from build123d import *

# Parameters (mm, degrees)
CUT_EXTRUDE1_REACH = 157.918
SKETCH2_R          = 19.05


with BuildPart() as part:
    # Sketch1 → Revolve1 (revolve)
    with BuildSketch(Plane.XY, mode=Mode.PRIVATE) as revolve1_sk:
        Polygon((0, 69.85), (0, 73.025), (-12.7, 73.025), (-51.194829198, 50.8), (-63.044090512, 50.8), (-63.044090512, 47.625), (-50.344090512, 47.625), (-11.849261314, 69.85), align=None)
    revolve(revolve1_sk.sketch.rotate(Axis((0, 0, 0), (-1, 0, 0)), 90), axis=Axis((0, 0, 0), (-1, 0, 0)))

    # Cut-Extrude1: up to this cone (the profile starts outside it)
    cut_extrude1_end = Plane(origin=(-34.795753, 0, 0), z_dir=(1, 0, 0)).offset(-98.037256223) * Cone(1e-06, 180.743597534, 313.057093071, align=(Align.CENTER, Align.CENTER, Align.MIN), mode=Mode.PRIVATE)
    # Sketch2 → Cut-Extrude1 (cut, up to the surface)
    with BuildSketch(Plane(origin=(-34.795752556, 0, 60.268011314), x_dir=(0.8660254037844378, 0, 0.5000000000000017), z_dir=(-0.5000000000000016, 0, 0.8660254037844377)), mode=Mode.PRIVATE) as cut_extrude1_sk1:
        with Locations(Location((0, 0, 0), (0, 0, 221.978854454))):
            Circle(SKETCH2_R)
    cut_extrude1_tool1 = extrude(cut_extrude1_sk1.sketch, amount=-CUT_EXTRUDE1_REACH, mode=Mode.PRIVATE) - cut_extrude1_end
    add(cut_extrude1_tool1.solids().sort_by_distance((-34.795753, 0, 60.268011))[0], mode=Mode.SUBTRACT)


solid = part.part
Source: CAD feature listing. Evaluate the final solid. Frame: model axes, mm. A direction names the side the tool comes from. Round coordinates to 2 decimals unless told otherwise and drop trailing zeros. Write each loop counter-clockwise with the first axis right and the second up, starting at its lowest first coordinate (ties: lowest second). Pieces come first, ordered by that corner, then holes. Notation, with made-up numbers: (7, -12.5) - (14, -12.5) arc R26 cw to (14, 11.5) - close; hole circle Ø10 at (5, -25.5). An arc over 180 degrees is marked (long way). Use CSV: the item, a comma, the result in double quotes. Start each with the question number.
(1) First-contact query: pin 1 Ø6 at (y, z) = (-9, 55) entering from -X; pin 2 Ø8 at (x, y) = (-27, -7.5) entering from +Z; pin 3 Ø8 at (x, y) = (-16, 55.5) entering from -Z; pin 4 Ø2 at (y, z) = (53.5, 36.5) entering from -X. Flat tips, straight axial feed; report the tip coordinate or a pass-through.
(2) Cut plane C-C, the plane y = 12. Give the number of separate pieces and of enclosed holes in the cut face, and give its area (3 significant figures).
(3) Mould query, pull axis Z, two halves, no side actions, for faces 3 (the face through (0, 38, 59)), 4 (the face through (-6.439, 64.786, -33.697)), 5 (the face through (-20.588, 12.107, 65.075)), 6 (the face through (-5.8, 68.2, 15.1)). Classes: pulls with the +Z half, pulls with the -Z half, needs draft (parallel to the pull), parting line crosses it, or undercut.
(4) Cut plane A-A, the plane z = 0. Return loops of the section in (x, y) (3 decimals), and give its area (3 significant figures).
(5) Material intervals for probe 1 along Y at (x, z) = (-5, 0) (3 decimals); probe 2 along Z at (x, y) = (-46, -16); probe 3 along Y at (x, z) = (-59, 0) (3 decimals), sorted ascending. Write a range as [from, to].
(6) Cut plane B-B, the plane x = -8.5. Return loops of the section in (y, z) (3 decimals).
(7) Set-up query: faces 1 (the face through (-57.202, 30.911, 40.313)), 2 (the face through (-47.94, -14.72, -46.75)). Return all of +Z, -Z, +X, -X, +Y, -Y with unobstructed straight access to the full face (end or side cutting, diameter ignored); none if empty.
Geometry says:
1,pin 1,"through"
1,pin 2,"z = -58.25"
1,pin 3,"z = -50.22"
1,pin 4,"x = -28.74"
2,separate pieces,"3"
2,enclosed holes,"0"
2,area,"352 mm²"
3,face 3,"needs draft"
3,face 4,"parting line crosses it"
3,face 5,"undercut"
3,face 6,"undercut"
4,outline,"(-63.044, -50.8) - (-51.195, -50.8) - (-12.7, -73.025) - (0, -73.025) - (0, -69.85) - (-11.849, -69.85) - (-50.344, -47.625) - (-63.044, -47.625) - close; (-63.044, 47.625) - (-50.344, 47.625) - (-11.849, 69.85) - (0, 69.85) - (0, 73.025) - (-12.7, 73.025) - (-51.195, 50.8) - (-63.044, 50.8) - close"
4,area,"438 mm²"
5,probe 1,"[-73.025, -69.85], [69.85, 73.025]"
5,probe 2,"[-51.36, -47.51], [47.51, 51.36]"
5,probe 3,"[-50.8, -47.625], [47.625, 50.8]"
6,outline,"circle Ø146.05 at (0, 0); hole circle Ø139.7 at (0, 0)"
7,face 1,"-X"
7,face 2,"+X"
